```python
from build123d import *

# Parameters (mm, degrees)
SKETCH1_R           = 4
BOSS_EXTRUDE1_DEPTH = 3
SKETCH2_W           = 11
SKETCH2_H           = 1
CUT_EXTRUDE1_DEPTH  = 13.4


with BuildPart() as part:
    # Sketch1 → Boss-Extrude1 (new body)
    with BuildSketch(Plane(origin=(0, 0, 0), x_dir=(1, 0, 0), z_dir=(0, 1, 0))):
        Polygon((43, 7.7), (43, -7.7), (6, -7.7), (6, -28.7), (5.499093619, -29.3), (4.500906381, -29.3), (4, -28.7), (3.499093619, -29.3), (2.500906381, -29.3), (2, -28.7), (1.499093619, -29.3), (0.500906381, -29.3), (0, -28.7), (0, 7.7), align=None)
        with Locations((16.5, 0)):
            Circle(SKETCH1_R, mode=Mode.SUBTRACT)
        with Locations((28.5, 0)):
            Circle(SKETCH1_R, mode=Mode.SUBTRACT)
    extrude(amount=BOSS_EXTRUDE1_DEPTH)

    # Sketch2 → Cut-Extrude1 (cut)
    with BuildSketch(Plane.XY.offset(7.7)):
        with Locations((16.5, 1.5)):
            Rectangle(SKETCH2_W, SKETCH2_H)
        with Locations((28.5, 1.5)):
            Rectangle(SKETCH2_W, SKETCH2_H)
    extrude(amount=-CUT_EXTRUDE1_DEPTH, mode=Mode.SUBTRACT)


solid = part.part
```
Geometry check sheet. Reference: the model listing, model coordinates, mm. A direction names the side the tool comes from. Coordinates: 2 decimals unless noted, no trailing zeros. Order: outer loops, then holes, each group sorted by start corner. A loop starts at its lowest first (then second) coordinate and runs counter-clockwise, first axis right, second up. Notation, with made-up numbers: M 76,37 L 88,37 A24 cw 88,68 Z; hole C 38,70 d2. An arc over 180 degrees is marked long. Answer as a JSON object with one key per item and string values.
Q1. Cross-section at A-A on z = 0. Record the cut outline in (x, y).
Results are:
{"outline": "M 0,0 L 12.5,0 L 12.5,1 L 11,1 L 11,2 L 12.5,2 L 12.5,3 L 0,3 Z; M 20.5,0 L 24.5,0 L 24.5,1 L 23,1 L 23,2 L 24.5,2 L 24.5,3 L 20.5,3 L 20.5,2 L 22,2 L 22,1 L 20.5,1 Z; M 32.5,0 L 43,0 L 43,3 L 32.5,3 L 32.5,2 L 34,2 L 34,1 L 32.5,1 Z"}
Q2. Release check for a two-part mould opening along X. For faces 1 (the cylindrical face through (12.504, 2.493, -0.176)), 2 (the flat face through (43, 1, 0)), 3 (the cylindrical face through (25.3, 2.5, 2.4)), 4 (the flat face through (0, 1, 11)) record: released by +X, released by -X, zero draft, split by the parting line, or undercut.
Results are:
{"face 1": "undercut", "face 2": "released by +X", "face 3": "undercut", "face 4": "released by -X"}
Q3. Tool access check on faces 5 (the flat face through (1, 1, 29.3)), 6 (the flat face through (30, 2, 4)), 7 (the flat face through (24.8, 0.8, 7.7)). Record the directions out of +Z, -Z, +X, -X, +Y, -Y that give a thin tool (end or side, any length) a straight path to the whole face; none if there is none.
Results are:
{"face 5": "+Z, +X, -X, +Y, -Y", "face 6": "+Z", "face 7": "+Z, +X, +Y, -Y"}
Q4. Cross-section at C-C on y = 2.55. Record the cut outline in (x, z).
Results are:
{"outline": "M 0,-7.7 L 43,-7.7 L 43,7.7 L 6,7.7 L 6,28.7 L 5.5,29.3 L 4.5,29.3 L 4,28.7 L 3.5,29.3 L 2.5,29.3 L 2,28.7 L 1.5,29.3 L 0.5,29.3 L 0,28.7 Z; hole C 16.5,0 d8; hole C 28.5,0 d8"}
Q5. Cross-section at B-B on x = 16.5. Record the cut outline in (y, z).
Results are:
{"outline": "M 0,-7.7 L 3,-7.7 L 3,-4 L 2,-4 L 2,-5.7 L 1,-5.7 L 1,-4 L 0,-4 Z; M 0,4 L 1,4 L 1,7.7 L 0,7.7 Z; M 2,4 L 3,4 L 3,7.7 L 2,7.7 Z"}
Q6. Scan lines: line 1 (X direction, y = 1.5, z = 7); line 2 (X direction, y = 2.3, z = 0); line 3 (Z direction, x = 16.5, y = 2.4). Record each from-to range of solid material in increasing order.
Results are:
{"line 1": "x = 0 to 11, 22 to 23, 34 to 43", "line 2": "x = 0 to 12.5, 20.5 to 24.5, 32.5 to 43", "line 3": "z = -7.7 to -4, 4 to 7.7"}
Q7. Depth check by flat-ended pin: pin 1 Ø0.8 at (x, y) = (16.5, 1.5) entering from +Z; pin 2 Ø0.9 at (x, y) = (26.5, 1) entering from +Z. Enter the tip coordinate at first touch or a pass-through.
Results are:
{"pin 1": "stops at z = -5.7", "pin 2": "stops at z = 7.7"}
Q8. Cross-section at D-D on x = 24. Record the cut outline in (y, z).
Results are:
{"outline": "M 0,-7.7 L 3,-7.7 L 3,7.7 L 2,7.7 L 2,-5.7 L 1,-5.7 L 1,7.7 L 0,7.7 Z"}
